from build123d import *

# Parameters (mm, degrees)
F0_R     = 17.5
F1_DEPTH = 5
F0_W     = 5
F0_H     = 1.25
F2_DEPTH = 2.5
F3_R     = 0.25
F4_R     = 0.5
F5_R     = 1.5


with BuildPart() as f1:
    # F0 (on Top) → F1 (new body)
    with BuildSketch(Plane.XY):
        Circle(F0_R)
        Polygon((-12.776, -2.25), (-12.776, 2.25), (-2.5, 2.25), (2.5, 2.25), (12.776, 2.25), (12.776, -2.25), (2.5, -2.25), (-2.5, -2.25), align=None, mode=Mode.SUBTRACT)
    extrude(amount=F1_DEPTH)

    # F0 (on Top) → F2 (join)
    with BuildSketch(Plane.XY):
        with Locations((0, 1.625)):
            Rectangle(F0_W, F0_H)
        with Locations((0, -1.625)):
            Rectangle(F0_W, F0_H)
    extrude(amount=F2_DEPTH)

    # F3
    f3_edges = [f1.edges().sort_by_distance(p)[0] for p in [
        (-2.5, -1, 1.25),
        (-2.5, -1.625, 2.5),
        (0, -1, 2.5),
        (2.5, -1.625, 2.5),
        (0, 1, 2.5),
        (2.5, 1.625, 2.5),
        (-2.5, 1.625, 2.5),
        (-2.5, 1, 1.25),
        (2.5, -1, 1.25),
        (2.5, 1, 1.25),
    ]]
    fillet(f3_edges, radius=F3_R)

    # F4
    f4_edges = [f1.edges().sort_by_distance(p)[0] for p in [
        (0, 2.25, 5),
        (12.776, 0, 5),
        (0, -2.25, 5),
        (-12.776, 0, 5),
    ]]
    fillet(f4_edges, radius=F4_R)

    # F5
    f5_edges = [f1.edges().sort_by_distance(p)[0] for p in [
        (-17.5, 0, 5),
    ]]
    fillet(f5_edges, radius=F5_R)


solid = f1.part
Can you work these out from the model? Positions are in its coordinate system, mm. A direction names the side the tool comes from. Coordinates: 2 decimals unless noted, no trailing zeros. Loops run counter-clockwise (first coordinate to the right, second up) from the corner with the lowest first, then second, coordinate; pieces in that order, holes last. Notation, with made-up numbers: M 21,77.25 L 80,77.25 A16 cw 80,82.25 Z; hole C 37.25,5.25 d9. An arc over 180 degrees is marked long. Return JSON: item names as keys, results as strings. Group by question number.
Item 1: I'm going to push flat-ended pins straight in: pin 1 Ø2 at (x, z) = (-3, 3) entering from -Y; pin 2 Ø1 at (x, z) = (8, 2.5) entering from +Y; pin 3 Ø0.8 at (x, y) = (-0.5, -2) entering from +Z. Where does each tip first touch, or does it pass through?
Item 2: Imagine slicing it at B-B (z = 1.3). Please give me the cut outline in (x, y), and give its area (3 significant figures).
Item 3: If I drill on L1, parallel to Y at x = -1.5, z = 3.3; L2, parallel to Y at x = 6, z = 2.85; L3, parallel to Z at x = -1, y = 1.5, over which ranges is the centre line in solid material (lowest first)? Write a range as from..to.
Item 4: Thinking about a two-plate mould opening in X: for faces 4 (the flat face through (2.5, 2, 1)), 5 (the flat face through (0, -4, 0)), 6 (the cylindrical face through (-13.887, -10.648, 1.726)), which applies, released by +X, released by -X, zero draft, split by the parting line, or undercut?
Item 5: Imagine slicing it at A-A (y = 0). Please give me the cut outline in (x, z), and give its area (3 significant figures).
Item 6: Imagine slicing it at C-C (x = 0). Please give me the cut outline in (y, z).
Item 7: On a 3-axis mill with a long thin cutter (end or side, diameter ignored), from which of +Z, -Z, +X, -X, +Y, -Y can I reach the whole of each face in a straight line? I mean faces 1 (the flat face through (0, -3, 5)), 2 (the flat face through (0, 2, 2.5)), 3 (the flat face through (2.5, -2, 1)). Say none if no direction works.
Verdict:
{
 "1": {"pin 1": "stops at y = -17.39", "pin 2": "stops at y = 15.81", "pin 3": "stops at z = 4.86"},
 "2": {"outline": "C 0,0 d35; hole M -12.78,-2.25 L -2.5,-2.25 L -2.5,-1.25 A0.25 cw -2.25,-1 L 2.25,-1 A0.25 cw 2.5,-1.25 L 2.5,-2.25 L 12.78,-2.25 L 12.78,2.25 L 2.5,2.25 L 2.5,1.25 A0.25 cw 2.25,1 L -2.25,1 A0.25 cw -2.5,1.25 L -2.5,2.25 L -12.78,2.25 Z", "area": "860 mm^2"},
 "3": {"L1": "y = -17.44..-2.25, 2.25..17.44", "L2": "y = -16.44..-2.25, 2.25..16.44", "L3": "z = 0..2.5"},
 "4": {"face 4": "undercut", "face 5": "zero draft", "face 6": "split by the parting line"},
 "5": {"outline": "M -17.5,0 L -12.78,0 L -12.78,4.5 A0.5 ccw -13.28,5 L -16,5 A1.5 ccw -17.5,3.5 Z; M 12.78,0 L 17.5,0 L 17.5,3.5 A1.5 ccw 16,5 L 13.28,5 A0.5 ccw 12.78,4.5 Z", "area": "46.2 mm^2"},
 "6": {"outline": "M -17.5,0 L -1,0 L -1,2.25 A0.25 ccw -1.25,2.5 L -2.25,2.5 L -2.25,4.5 A0.5 ccw -2.75,5 L -16,5 A1.5 ccw -17.5,3.5 Z; M 1,0 L 17.5,0 L 17.5,3.5 A1.5 ccw 16,5 L 2.75,5 A0.5 ccw 2.25,4.5 L 2.25,2.5 L 1.25,2.5 A0.25 ccw 1,2.25 Z"},
 "7": {"face 1": "+Z, +X, -X, +Y, -Y", "face 2": "+Z", "face 3": "+Z, -Z"}
}
